Can you work these out from the model? Positions are in its coordinate system, mm. Face numbers are marked on the shaded views. A direction names the side the tool comes from. Coordinates: 2 decimals unless noted, no trailing zeros. Write each loop counter-clockwise with the first axis right and the second up, starting at its lowest first coordinate (ties: lowest second). Pieces come first, ordered by that corner, then holes. Notation, with made-up numbers: (34.5, -15.75) -> (61.5, -15.75) arc R18 cw to (61.5, 18.25) -> close; hole circle Ø9 at (-30, 13.5). An arc over 180 degrees is marked (long way). Use one line per item in the form item = value.
```python
from build123d import *

# Parameters (mm, degrees)
SKETCH1_R                                      = 47
BOSS_EXTRUDE1_DEPTH                            = 5.08
CSK_FOR_M8_FLAT_HEAD_MACHINE_SCREW1_AT_2_COUNT = 2
CSK_FOR_M8_FLAT_HEAD_MACHINE_SCREW1_AT_2_PITCH = 37.5
CSK_FOR_M8_FLAT_HEAD_MACHINE_SCREW1_AT_3_COUNT = 2
CSK_FOR_M8_FLAT_HEAD_MACHINE_SCREW1_AT_3_PITCH = 37.5
CSK_FOR_M8_FLAT_HEAD_MACHINE_SCREW1_AT_4_COUNT = 2
CSK_FOR_M8_FLAT_HEAD_MACHINE_SCREW1_AT_4_PITCH = 64.951905284
CSK_FOR_M8_FLAT_HEAD_MACHINE_SCREW1_AT_5_COUNT = 2
CSK_FOR_M8_FLAT_HEAD_MACHINE_SCREW1_AT_5_PITCH = 75
CSK_FOR_M8_FLAT_HEAD_MACHINE_SCREW1_AT_6_COUNT = 2
CSK_FOR_M8_FLAT_HEAD_MACHINE_SCREW1_AT_6_PITCH = 64.951905284
SKETCH11_R                                     = 27.94
BOSS_EXTRUDE2_DEPTH                            = 7.62


with BuildPart() as part:
    # Sketch1 → Boss-Extrude1 (new body)
    with BuildSketch(Plane.XY):
        Circle(SKETCH1_R)
        with BuildLine():
            Line((-4.7625, 20.354769843), (-4.7625, 15.274769843))
            ThreePointArc((-4.7625, 15.274769843), (0, -16), (4.7625, 15.274769843))
            Line((4.7625, 15.274769843), (4.7625, 20.354769843))
            Line((4.7625, 20.354769843), (-4.7625, 20.354769843))
        make_face(mode=Mode.SUBTRACT)
    extrude(amount=BOSS_EXTRUDE1_DEPTH)

    # Sketch10 → CSK for M8 Flat Head Machine Screw1 (revolve, cut)
    with BuildSketch(Plane(origin=(-10.251484687, 36.071554745, 5.08), x_dir=(0, -1, 0), z_dir=(1, 0, 0))):
        Polygon((0, 0), (0, 5.08), (4.5, 5.08), (4.5, 4.15), (8.65, 0), align=None)
    csk_for_m8_flat_head_machine_screw1 = revolve(axis=Axis((-10.251484687, 36.071554745, 11.43), (0, 0, -1)), mode=Mode.SUBTRACT)

    # CSK for M8 Flat Head Machine Screw1 at 2: CSK for M8 Flat Head Machine Screw1 ×2
    with Locations(*[Vector(0.969723336, -0.244206166, 0) * (i * CSK_FOR_M8_FLAT_HEAD_MACHINE_SCREW1_AT_2_PITCH) for i in range(1, CSK_FOR_M8_FLAT_HEAD_MACHINE_SCREW1_AT_2_COUNT)]):
        add(csk_for_m8_flat_head_machine_screw1, mode=Mode.SUBTRACT)

    # CSK for M8 Flat Head Machine Screw1 at 3: CSK for M8 Flat Head Machine Screw1 ×2
    with Locations(*[Vector(-0.696350411, -0.717701961, 0) * (i * CSK_FOR_M8_FLAT_HEAD_MACHINE_SCREW1_AT_3_PITCH) for i in range(1, CSK_FOR_M8_FLAT_HEAD_MACHINE_SCREW1_AT_3_COUNT)]):
        add(csk_for_m8_flat_head_machine_screw1, mode=Mode.SUBTRACT)

    # CSK for M8 Flat Head Machine Screw1 at 4: CSK for M8 Flat Head Machine Screw1 ×2
    with Locations(*[Vector(0.717701961, -0.696350411, 0) * (i * CSK_FOR_M8_FLAT_HEAD_MACHINE_SCREW1_AT_4_PITCH) for i in range(1, CSK_FOR_M8_FLAT_HEAD_MACHINE_SCREW1_AT_4_COUNT)]):
        add(csk_for_m8_flat_head_machine_screw1, mode=Mode.SUBTRACT)

    # CSK for M8 Flat Head Machine Screw1 at 5: CSK for M8 Flat Head Machine Screw1 ×2
    with Locations(*[Vector(0.273372925, -0.961908127, 0) * (i * CSK_FOR_M8_FLAT_HEAD_MACHINE_SCREW1_AT_5_PITCH) for i in range(1, CSK_FOR_M8_FLAT_HEAD_MACHINE_SCREW1_AT_5_COUNT)]):
        add(csk_for_m8_flat_head_machine_screw1, mode=Mode.SUBTRACT)

    # CSK for M8 Flat Head Machine Screw1 at 6: CSK for M8 Flat Head Machine Screw1 ×2
    with Locations(*[Vector(-0.244206166, -0.969723336, 0) * (i * CSK_FOR_M8_FLAT_HEAD_MACHINE_SCREW1_AT_6_PITCH) for i in range(1, CSK_FOR_M8_FLAT_HEAD_MACHINE_SCREW1_AT_6_COUNT)]):
        add(csk_for_m8_flat_head_machine_screw1, mode=Mode.SUBTRACT)

    # Sketch11 → Boss-Extrude2 (add)
    with BuildSketch(Plane(origin=(0, 0, 0), x_dir=(-1, 0, 0), z_dir=(0, 0, -1))):
        Circle(SKETCH11_R)
        with BuildLine():
            ThreePointArc((4.7625, 15.274769843), (0, -16), (-4.7625, 15.274769843))
            Line((-4.7625, 15.274769843), (-4.7625, 20.354769843))
            Line((-4.7625, 20.354769843), (4.7625, 20.354769843))
            Line((4.7625, 20.354769843), (4.7625, 15.274769843))
        make_face(mode=Mode.SUBTRACT)
    extrude(amount=BOSS_EXTRUDE2_DEPTH)


solid = part.part
```
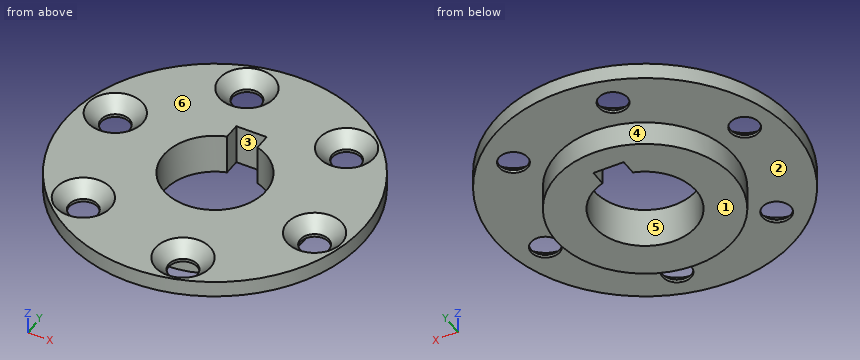
Q1. Will these pins go through, and if not, where does the flat tip stop? pin 1 (6 mm diameter, centred on x = 28, y = -14.5, fed in from -Z); pin 2 (3 mm diameter, centred on x = -3, z = 2, fed in from -Y); pin 3 (2.5 mm diameter, centred on y = 19, z = -1, fed in from +X).
Return value:
pin_1 = 0
pin_2 = -46.98
pin_3 = 43.31
Q2. Suppose I cut it at A-A (x = 0). Write out the boundary of the cut face in (y, z).
Return value:
outline = (-47, 0) -> (-27.94, 0) -> (-27.94, -7.62) -> (-16, -7.62) -> (-16, 5.08) -> (-47, 5.08) -> close; (20.35, -7.62) -> (27.94, -7.62) -> (27.94, 0) -> (47, 0) -> (47, 5.08) -> (20.35, 5.08) -> close
Q3. Suppose I cut it at B-B (z = -2.75). Write out the boundary of the cut face in (x, y), then the cut area to 3 significant figures.
Return value:
outline = circle Ø55.88 at (0, 0); hole (-4.76, 15.27) arc R16 ccw (long way) to (4.76, 15.27) -> (4.76, 20.35) -> (-4.76, 20.35) -> close
area = 1,600 mm2
Q4. Thinking about a two-plate mould opening in X: for the marked faces 4, 5 and 6, which applies, released by +X, released by -X, zero draft, split by the parting line, or undercut?
Return value:
face_4 = split by the parting line
face_5 = undercut
face_6 = zero draft
Q5. For the marked faces 1, 2 and 3, which set-ups out of +Z, -Z, +X, -X, +Y, -Y let a thin tool reach every point of the face, with its end or its side?
Return value:
face_1 = -Z, +X, -X, +Y, -Y
face_2 = -Z
face_3 = +Z, -Z
Q6. If I drill on line 1 (X direction, y = 10, z = 1.5); line 2 (X direction, y = 13, z = 1.5); line 3 (X direction, y = 0.5, z = -4.5), over which ranges is the centre line in solid material (lowest first)? Write a range as from..to.
Return value:
line_1 = -45.92..-41.36, -31.37..-12.49, 12.49..45.92
line_2 = -45.17..-39.67, -33.06..-9.33, 9.33..45.17
line_3 = -27.94..-15.99, 15.99..27.94
Q7. Suppose I cut it at C-C (x = 12.5). Give the number of separate pieces and of enclosed holes in the cut face, then the cut area to 3 significant figures.
Return value:
separate_pieces = 3
enclosed_holes = 0
area = 529 mm2
